Design review of the part built by this model. Coordinates are the model's own, in mm. A direction names the side the tool comes from. Round coordinates to 2 decimals unless told otherwise and drop trailing zeros. Loops run counter-clockwise (first coordinate to the right, second up) from the corner with the lowest first, then second, coordinate; pieces in that order, holes last. Notation, with made-up numbers: (-32, 35) - (-6, 35) arc R20 cw to (-6, 51) - close; hole circle Ø2 at (39, 21). An arc over 180 degrees is marked (long way). One line per question, with ' | ' between items. Start each with the question number.
from build123d import *

# Parameters (mm, degrees)
BOSS_EXTRUDE1_DEPTH = 57.15
BOSS_EXTRUDE2_DEPTH = 57.15
CUT_EXTRUDE1_REACH  = 59.15
SKETCH4_R           = 19.05
SKETCH5_R           = 3.175
CUT_EXTRUDE2_DEPTH  = 25.4
SKETCH7_R           = 3.175
CUT_EXTRUDE3_DEPTH  = 58.15


with BuildPart() as part:
    # Sketch2 → Boss-Extrude1 (new body)
    with BuildSketch(Plane(origin=(0, 0, 0), x_dir=(0, 0, -1), z_dir=(1, 0, 0))):
        with BuildLine():
            Line((45.71235962, 13.716504708), (-1.91264038, 13.716504708))
            ThreePointArc((-1.91264038, 13.716504708), (-8.647832471, 10.926696799), (-11.43764038, 4.191504708))
            Line((-11.43764038, 4.191504708), (-11.43764038, -43.433495292))
            Line((-11.43764038, -43.433495292), (4.43735962, -43.433495292))
            Line((4.43735962, -43.433495292), (4.43735962, -2.158495292))
            Line((4.43735962, -2.158495292), (45.71235962, -2.158495292))
            Line((45.71235962, -2.158495292), (45.71235962, 13.716504708))
        make_face()
    extrude(amount=BOSS_EXTRUDE1_DEPTH)

    # Sketch3 → Boss-Extrude2 (add)
    with BuildSketch(Plane(origin=(0, 0, 0), x_dir=(0, 0, -1), z_dir=(1, 0, 0))):
        with BuildLine():
            Line((4.43735962, -5.333495292), (4.43735962, -2.158495292))
            Line((4.43735962, -2.158495292), (7.61235962, -2.158495292))
            ThreePointArc((7.61235962, -2.158495292), (5.36729559, -3.088431262), (4.43735962, -5.333495292))
        make_face()
    extrude(amount=BOSS_EXTRUDE2_DEPTH)

    # Sketch4 → Cut-Extrude1 (cut, up to next)
    with BuildSketch(Plane(origin=(0, 13.716504708, 0), x_dir=(1, 0, 0), z_dir=(0, 1, 0)), mode=Mode.PRIVATE) as cut_extrude1_sk1:
        with Locations((28.575, 45.71235962)):
            Circle(SKETCH4_R)
    cut_extrude1_tool1 = extrude(cut_extrude1_sk1.sketch, amount=-CUT_EXTRUDE1_REACH, mode=Mode.PRIVATE) & part.part
    add(cut_extrude1_tool1.solids().sort_by_distance((28.575, 13.716505, -45.71236))[0], mode=Mode.SUBTRACT)

    # Sketch5 → Cut-Extrude2 (cut)
    with BuildSketch(Plane(origin=(41.275, 0, 0), x_dir=(0, 0, -1), z_dir=(1, 0, 0))):
        with BuildLine():
            Line((7.61235962, -2.158495292), (7.61235962, 13.716504708))
            Line((7.61235962, 13.716504708), (-1.91264038, 13.716504708))
            ThreePointArc((-1.91264038, 13.716504708), (-8.647832471, 10.926696799), (-11.43764038, 4.191504708))
            Line((-11.43764038, 4.191504708), (-11.43764038, -2.158495292))
            Line((-11.43764038, -2.158495292), (-11.43764038, -5.333495292))
            Line((-11.43764038, -5.333495292), (4.43735962, -5.333495292))
            ThreePointArc((4.43735962, -5.333495292), (5.36729559, -3.088431262), (7.61235962, -2.158495292))
        make_face()
        with Locations((-1.91264038, 4.191504708)):
            Circle(SKETCH5_R, mode=Mode.SUBTRACT)
    extrude(amount=-CUT_EXTRUDE2_DEPTH, mode=Mode.SUBTRACT)

    # Sketch7 → Cut-Extrude3 (cut, through all)
    with BuildSketch(Plane(origin=(57.15, 0, 0), x_dir=(0, 0, -1), z_dir=(1, 0, 0))):
        with Locations((-1.91264038, 4.191504708)):
            Circle(SKETCH7_R)
    extrude(amount=-CUT_EXTRUDE3_DEPTH, mode=Mode.SUBTRACT)


solid = part.part
1. The part is to be moulded in two halves that separate along Z. For faces 1 (the face through (49.32, 6.34, 4.25)), 2 (the face through (5, 6, -45.712)), 3 (the face through (15.875, 4, -2)), say which applies: pulls with the +Z half, pulls with the -Z half, needs draft (parallel to the pull), parting line crosses it, or undercut.
2. Clearance check with flat-ended pins moving along their axes: P1, Ø12, axis at x = 35, y = 7, coming from the -Z side; P2, Ø12, axis at x = 46.5, y = -13, coming from the -Z side; P3, Ø8, axis at x = 34, y = 3.5, coming from the +Z side. State where each tip first meets the part, or that it passes through.
3. Take a section at B-B, the plane y = 2.5. Give the boundary of the cut face in (x, z) (3 decimals).
4. Take a section at A-A, the plane z = -35.5. Give the boundary of the cut face in (x, y).
5. To check wall thickness, follow line 1 along Y through (x, z) = (9, -19); line 2 along Z through (x, y) = (9, -28); line 3 along Z through (x, y) = (49, 7). State the ranges of each line that lie inside material, in increasing order.
6. Machinability: for faces 4 (the face through (41.275, 4, -2)), 5 (the face through (29, -5.333, 4)), 6 (the face through (29, 6, -7.612)), 7 (the face through (28, -25, -4.437)), which of the approach directions +Z, -Z, +X, -X, +Y, -Y give a long, thin tool a straight path to every point of the face, cutting with its end or side? Answer none if there is none.
Answer list:
1) face 1: undercut | face 2: pulls with the -Z half | face 3: needs draft
2) P1: stops at z = -31.27 | P2: stops at z = -4.44 | P3: stops at z = -7.61
3) outline: (0, -45.712) - (9.525, -45.712) arc R19.05 cw to (47.625, -45.712) - (57.15, -45.712) - (57.15, -0.774) - (41.275, -0.774) - (41.275, -7.612) - (15.875, -7.612) - (15.875, -0.774) - (0, -0.774) - close; (0, 4.6) - (15.875, 4.6) - (15.875, 11.438) - (0, 11.438) - close; (41.275, 4.6) - (57.15, 4.6) - (57.15, 11.438) - (41.275, 11.438) - close
4) outline: (0, -2.16) - (12.49, -2.16) - (12.49, 13.72) - (0, 13.72) - close; (44.66, -2.16) - (57.15, -2.16) - (57.15, 13.72) - (44.66, 13.72) - close
5) line 1: y = -2.16 to 13.72 | line 2: z = -4.44 to 11.44 | line 3: z = -45.71 to 0.43, 3.39 to 11.01
6) face 4: +Z, +Y | face 5: +Z, -Z, +Y | face 6: +Z, +Y, -Y | face 7: -Z, +X, -X, -Y
